Can you work these out from the model? Positions are in its coordinate system, mm. A direction names the side the tool comes from. Give positions to 0.01 mm unless a question says otherwise; leave off trailing zeros. Order: outer loops, then holes, each group sorted by start corner. A loop starts at its lowest first (then second) coordinate and runs counter-clockwise, first axis right, second up. Notation, with made-up numbers: M 50,10.25 L 77,10.25 A11 cw 77,24.25 Z; hole C 35,-17.75 d7. An arc over 180 degrees is marked long. Use one line per item in the form item = value. Start each with the question number.
1. I want a section at B-B, the plane y = -62.5. Count the separate pieces of the cut face and the enclosed holes in it, and give its area (3 significant figures).
2. For faces 1 (the face through (-97.698, -50.053, 47.386)), 2 (the face through (-2, -123, -36.467)), 3 (the face through (-97, -124.55, -83)), 4 (the face through (120, -76, -1)), which set-ups out of +Z, -Z, +X, -X, +Y, -Y let a thin tool reach every point of the face, with its end or its side?
3. We'd pull the mould along Z, two halves only. Please class faces 5 (the face through (-98, -76, 60.668)), 6 (the face through (-97, -123.45, -83)), 7 (the face through (-2, -48, -87.5)): +Z half, -Z half, draft (parallel to the pull), parting line (faces both ways), or undercut.
4. Will these pins go through, and if not, where does the flat tip stop? P1, Ø2, axis at x = -49.5, z = 15, coming from the -Y side; P2, Ø6, axis at x = -42, y = -94, coming from the -Z side.
5. I want a section at C-C, the plane z = 65. List the corners of the cut face in (x, y) for me.
6. I need wall thicknesses on L1, parallel to X at y = -103, z = 41.5; L2, parallel to X at y = -47.5, z = -66; L3, parallel to Z at x = 104, y = -83. Which ranges of each line are inside material? Lowest first, please.
7. I want a section at D-D, the plane y = -78.5. List the corners of the cut face in (x, z) for me, and give its area (3 significant figures).
8. I want a section at A-A, the plane x = 57. List the corners of the cut face in (y, z) for me.
```python
from build123d import *

# Parameters (mm, degrees)
SKETCH1_W               = 250
SKETCH1_H               = 175
BOSS_EXTRUDE1_DEPTH     = 125
SKETCH2_W               = 240
SKETCH2_H               = 165
CUT_EXTRUDE1_DEPTH      = 120
SKETCH3_W               = 40.1
SKETCH3_H               = 165
CUT_EXTRUDE2_DEPTH      = 198.246672976
SKETCH6_W               = 250
SKETCH6_H               = 175
BOSS_EXTRUDE2_DEPTH     = 5
SKETCH7_W               = 205
SKETCH7_H               = 30
PIANO_PLUG_DEPTH        = 5
ARM_HOLE_REACH          = 199.247
SKETCH8_W               = 50
SKETCH8_H               = 180
BOSS_EXTRUDE8_REACH     = 216.001
SKETCH4_R               = 6
MAIN_SHAFT_HOLE_DEPTH   = 293.884362846
CUT_EXTRUDE8_DEPTH      = 16
CUT_EXTRUDE8_DEPTH_BACK = 33
SKETCH10_R              = 20
BOTTOM_OPEN_DEPTH       = 28
BOTTOM_OPEN_DEPTH_BACK  = 21
SKETCH11_W              = 230
SKETCH11_H              = 155
SKETCH12_W              = 41.033462292
SKETCH12_H              = 5
BOSS_EXTRUDE4_DEPTH     = 233
SKETCH13_W              = 7.5
SKETCH13_H              = 80
BOSS_EXTRUDE5_DEPTH     = 49
SKETCH14_W              = 44.113211518
SKETCH14_H              = 5
BOSS_EXTRUDE6_DEPTH     = 21
FILLET2_R               = 5
SKETCH16_R              = 2.5
SKETCH16_W              = 20
SKETCH16_H              = 42
SERVO_PLUG_HOLE_DEPTH   = 106
SKETCH17_W              = 49.113211518
SKETCH17_H              = 12.164138601
BOSS_EXTRUDE7_DEPTH     = 23
SKETCH19_W              = 10.1
SKETCH19_H              = 5.6
CUT_EXTRUDE9_DEPTH      = 2
SKETCH21_W              = 10.1
SKETCH21_H              = 1.1
CUT_EXTRUDE10_DEPTH     = 10


with BuildPart() as part:
    # Sketch1 → Boss-Extrude1 (new body)
    with BuildSketch(Plane(origin=(0, 0, 0), x_dir=(1, 0, 0), z_dir=(0, 1, 0))):
        Rectangle(SKETCH1_W, SKETCH1_H)
    extrude(amount=-BOSS_EXTRUDE1_DEPTH)

    # Sketch2 → Cut-Extrude1 (cut)
    with BuildSketch(Plane.XZ.offset(125)):
        Rectangle(SKETCH2_W, SKETCH2_H)
    extrude(amount=-CUT_EXTRUDE1_DEPTH, mode=Mode.SUBTRACT)

    # Sketch3 → Cut-Extrude2 (cut, through all)
    with BuildSketch(Plane(origin=(0, 0, 0), x_dir=(1, 0, 0), z_dir=(0, 1, 0))):
        Rectangle(SKETCH3_W, SKETCH3_H)
    extrude(amount=-CUT_EXTRUDE2_DEPTH, mode=Mode.SUBTRACT)

    # Sketch6 → Boss-Extrude2 (add)
    with BuildSketch(Plane.XZ.offset(125)):
        Rectangle(SKETCH6_W, SKETCH6_H)
    extrude(amount=-BOSS_EXTRUDE2_DEPTH)

    # Sketch7 → Piano Plug (cut)
    with BuildSketch(Plane(origin=(0, 0, -87.5), x_dir=(-1, 0, 0), z_dir=(0, 0, -1))):
        with Locations((0, -105)):
            Rectangle(SKETCH7_W, SKETCH7_H)
    extrude(amount=-PIANO_PLUG_DEPTH, mode=Mode.SUBTRACT)

    # Arm Hole: up to this face of the body (flat: up to its plane)
    arm_hole_end = Plane(part.part.faces().sort_by_distance((0, -120, -2.144615385))[0])
    # Sketch8 → Arm Hole (cut, up to the picked face)
    with BuildSketch(Plane(origin=(0, 0, 0), x_dir=(1, 0, 0), z_dir=(0, 1, 0)), mode=Mode.PRIVATE) as arm_hole_sk1:
        with Locations((-0.05, -2.5)):
            Rectangle(SKETCH8_W, SKETCH8_H)
    arm_hole_tool1 = split(extrude(arm_hole_sk1.sketch, amount=-ARM_HOLE_REACH, mode=Mode.PRIVATE), bisect_by=arm_hole_end, keep=Keep.BOTH, mode=Mode.PRIVATE)
    add(arm_hole_tool1.solids().sort_by(Axis((-0.05, 0, 2.5), (0, -1, 0)))[0], mode=Mode.SUBTRACT)

    # Sketch9 → Boss-Extrude8 (add, up to next)
    with BuildSketch(Plane(origin=(-25.05, 0, 0), x_dir=(0, 0, -1), z_dir=(1, 0, 0)), mode=Mode.PRIVATE) as boss_extrude8_sk1:
        Polygon((87.5, 0), (87.5, -90), (82.5, -90), (82.5, -5), (0, -5), (0, 0), align=None)
    boss_extrude8_tool1 = extrude(boss_extrude8_sk1.sketch, amount=BOSS_EXTRUDE8_REACH, mode=Mode.PRIVATE) - part.part
    add(boss_extrude8_tool1.solids().sort_by_distance((-25.05, -45, -86.244761))[0])

    # Sketch4 → Main Shaft Hole (cut, through all)
    with BuildSketch(Plane.ZY.offset(125)):
        with Locations((0, -62.5)):
            Circle(SKETCH4_R)
    extrude(amount=-MAIN_SHAFT_HOLE_DEPTH, mode=Mode.SUBTRACT)

    # Sketch10 → Cut-Extrude8 (cut, two sides: drawn at the far end of the back side and taken through both)
    with BuildSketch(Plane.ZY.offset(125).offset(-CUT_EXTRUDE8_DEPTH_BACK)):
        with Locations((50.8, -62.5)):
            Circle(SKETCH10_R)
    extrude(amount=CUT_EXTRUDE8_DEPTH + CUT_EXTRUDE8_DEPTH_BACK, mode=Mode.SUBTRACT)

    # Sketch11 → Bottom Open (cut, two sides: drawn at the far end of the back side and taken through both)
    with BuildSketch(Plane(origin=(0, -125, 0), x_dir=(-1, 0, 0), z_dir=(0, -1, 0)).offset(-BOTTOM_OPEN_DEPTH_BACK)):
        Rectangle(SKETCH11_W, SKETCH11_H)
    extrude(amount=BOTTOM_OPEN_DEPTH + BOTTOM_OPEN_DEPTH_BACK, mode=Mode.SUBTRACT)

    # Sketch12 → Boss-Extrude4 (add)
    with BuildSketch(Plane(origin=(-115, 0, 0), x_dir=(0, 0, -1), z_dir=(1, 0, 0))):
        with Locations((56.983268854, -122.5)):
            Rectangle(SKETCH12_W, SKETCH12_H)
    extrude(amount=BOSS_EXTRUDE4_DEPTH)

    # Sketch13 → Boss-Extrude5 (add)
    with BuildSketch(Plane(origin=(0, 0, 82.5), x_dir=(-1, 0, 0), z_dir=(0, 0, -1))):
        with Locations((97.75, -80)):
            Rectangle(SKETCH13_W, SKETCH13_H)
    extrude(amount=BOSS_EXTRUDE5_DEPTH)

    # Sketch14 → Boss-Extrude6 (add)
    with BuildSketch(Plane(origin=(-115, 0, 0), x_dir=(0, 0, -1), z_dir=(1, 0, 0))):
        with Locations((-55.443394241, -122.5)):
            Rectangle(SKETCH14_W, SKETCH14_H)
    extrude(amount=BOSS_EXTRUDE6_DEPTH)

    # Fillet2
    # the kernel refuses this fillet: 5 mm, written as the material it adds along each edge
    with BuildSketch(Plane(origin=(-101.5, -120, 33.5), x_dir=(0, 1, 0), z_dir=(1, 0, 0))) as fillet2_piece_1:
        with BuildLine():
            CenterArc((1.057968965, -5), FILLET2_R, 90, 12.215768954)
            Line((0, -0.113211518), (-0.021159379, -0.015475748))
            ThreePointArc((-0.021159379, -0.015475748), (-0.1, -0.056605759), (-0.1, 0))
            Line((-0.1, 0), (0, 0.1))
            Line((0, 0.1), (1.057968965, 0.1))
            Line((1.057968965, 0.1), (1.057968965, 0))
        make_face()
    extrude(amount=7.5)

    # Sketch16 → Servo Plug Hole (cut)
    with BuildSketch(Plane(origin=(0, 0, 0), x_dir=(0, 0, -1), z_dir=(1, 0, 0))):
        with Locations((-45.543439041, -51.74216133)):
            Circle(SKETCH16_R)
        with Locations((-55.793439041, -51.74216133)):
            Circle(SKETCH16_R)
        with Locations((-50.668439041, -75.74216133)):
            Rectangle(SKETCH16_W, SKETCH16_H)
        with Locations((-45.543439041, -99.74216133)):
            Circle(SKETCH16_R)
        with Locations((-55.793439041, -99.74216133)):
            Circle(SKETCH16_R)
    extrude(amount=-SERVO_PLUG_HOLE_DEPTH, mode=Mode.SUBTRACT)

    # Sketch17 → Boss-Extrude7 (add)
    with BuildSketch(Plane.ZY.offset(101.5)):
        with Locations((57.943394241, -113.9179307)):
            Rectangle(SKETCH17_W, SKETCH17_H)
    extrude(amount=BOSS_EXTRUDE7_DEPTH)

    # Sketch19 → Cut-Extrude9 (cut)
    with BuildSketch(Plane(origin=(0, -120, 0), x_dir=(1, 0, 0), z_dir=(0, 1, 0))):
        with Locations((97.45, 49.8)):
            Rectangle(SKETCH19_W, SKETCH19_H)
        with Locations((-97.45, 49.8)):
            Rectangle(SKETCH19_W, SKETCH19_H)
        with Locations((0, 49.8)):
            Rectangle(SKETCH19_W, SKETCH19_H)
    extrude(amount=-CUT_EXTRUDE9_DEPTH, mode=Mode.SUBTRACT)

    # Sketch21 → Cut-Extrude10 (cut)
    with BuildSketch(Plane(origin=(0, 0, -87.5), x_dir=(-1, 0, 0), z_dir=(0, 0, -1))):
        with Locations((-97.45, -124)):
            Rectangle(SKETCH21_W, SKETCH21_H)
        with Locations((97.45, -124)):
            Rectangle(SKETCH21_W, SKETCH21_H)
        with Locations((0, -124)):
            Rectangle(SKETCH21_W, SKETCH21_H)
    extrude(amount=-CUT_EXTRUDE10_DEPTH, mode=Mode.SUBTRACT)


solid = part.part
```
Check result:
q1.separate_pieces = 5
q1.enclosed_holes = 0
q1.area = 3,800 mm2
q2.face_1 = -X
q2.face_2 = -Y
q2.face_3 = -Z
q2.face_4 = none
q3.face_5 = undercut
q3.face_6 = draft
q3.face_7 = -Z half
q4.P1 = -5
q4.P2 = 82.5
q5.outline = M -125,-125 L -94,-125 L -94,-40 L -101.5,-40 L -101.5,-107.84 L -120,-107.84 L -120,-76.58 L -125,-76.58 Z; M -125,-48.42 L -120,-48.42 L -120,-5 L -25.05,-5 L -25.05,0 L -125,0 Z; M 24.95,-5 L 120,-5 L 120,-120 L 115,-120 L 115,-125 L 125,-125 L 125,0 L 24.95,0 Z
q6.L1 = -125 to -120, -101.5 to -94, 120 to 125
q6.L2 = -125 to -120, 120 to 125
q6.L3 = -87.5 to -82.5, 82.5 to 87.5
q7.outline = M -125,-87.5 L 125,-87.5 L 125,87.5 L 24.95,87.5 L 24.95,82.5 L 120,82.5 L 120,-82.5 L -120,-82.5 L -120,38.8 L -125,38.8 Z; M -125,62.8 L -120,62.8 L -120,82.5 L -101.5,82.5 L -101.5,60.67 L -94,60.67 L -94,82.5 L -25.05,82.5 L -25.05,87.5 L -125,87.5 Z; M -101.5,33.5 L -94,33.5 L -94,40.67 L -101.5,40.67 Z
q7.area = 4,000 mm2
q8.outline = M -125,-87.5 L -120,-87.5 L -120,-36.47 L -125,-36.47 Z; M -125,77.5 L -120,77.5 L -120,82.5 L -5,82.5 L -5,-82.5 L -90,-82.5 L -90,-87.5 L 0,-87.5 L 0,87.5 L -125,87.5 Z
